```python
from build123d import *

# Parameters (mm, degrees)
SKETCH021_W             = 51.5
SKETCH021_H             = 3
SKETCH021_W_2           = 3
SKETCH021_H_2           = 51.5
PAD014_DEPTH            = 1.6
SKETCH022_R             = 3
PAD015_DEPTH            = 2.6
HOLE_D                  = 3.4
HOLE_DEPTH              = 25
HOLE_CSINK_D            = 6.7
HOLE_CSINK_ANGLE        = 90
BODY005_PLACEMENT_ANGLE = 180


with BuildPart() as part:
    # Sketch021 → Pad014 (new body)
    with BuildSketch(Plane.XY):
        with BuildLine():
            ThreePointArc((-43, 41), (-46.535534, 39.535534), (-48, 36))
            Line((-48, -36), (-48, 36))
            ThreePointArc((-48, -36), (-46.535534, -39.535534), (-43, -41))
            Line((43, -41), (-43, -41))
            ThreePointArc((43, -41), (46.535534, -39.535534), (48, -36))
            Line((48, 36), (48, -36))
            ThreePointArc((48, 36), (46.535534, 39.535534), (43, 41))
            Line((-43, 41), (43, 41))
        make_face()
        with Locations((0, 22)):
            Rectangle(SKETCH021_W, SKETCH021_H, mode=Mode.SUBTRACT)
        with Locations((0, -22)):
            Rectangle(SKETCH021_W, SKETCH021_H, mode=Mode.SUBTRACT)
        with Locations((-36.5, 0)):
            Rectangle(SKETCH021_W_2, SKETCH021_H_2, mode=Mode.SUBTRACT)
        with Locations((36.5, 0)):
            Rectangle(SKETCH021_W_2, SKETCH021_H_2, mode=Mode.SUBTRACT)
    extrude(amount=PAD014_DEPTH)

    # Sketch022 → Pad015 (join)
    with BuildSketch(Plane.XY):
        with Locations((-44, 37)):
            Circle(SKETCH022_R)
        with Locations((12, 37)):
            Circle(SKETCH022_R)
        with Locations((44, 37)):
            Circle(SKETCH022_R)
        with Locations((44, -37)):
            Circle(SKETCH022_R)
        with Locations((12, -37)):
            Circle(SKETCH022_R)
        with Locations((-44, -37)):
            Circle(SKETCH022_R)
    extrude(amount=PAD015_DEPTH)

    # Hole
    with Locations(Plane(origin=(0, 0, 0), x_dir=(1, 0, 0), z_dir=(0, 0, -1))):
        with Locations((-44, -37), (12, -37), (44, -37), (44, 37), (12, 37), (-44, 37)):
            CounterSinkHole(HOLE_D / 2, HOLE_CSINK_D / 2, depth=HOLE_DEPTH, counter_sink_angle=HOLE_CSINK_ANGLE)


with BuildPart() as part_1:
    # Body005 placement: moved
    add(part.part.moved(Location((0, 0, 80.3))).rotate(Axis((0, 0, 80.3), (1, 0, 0)), BODY005_PLACEMENT_ANGLE))


solid = part_1.part
```
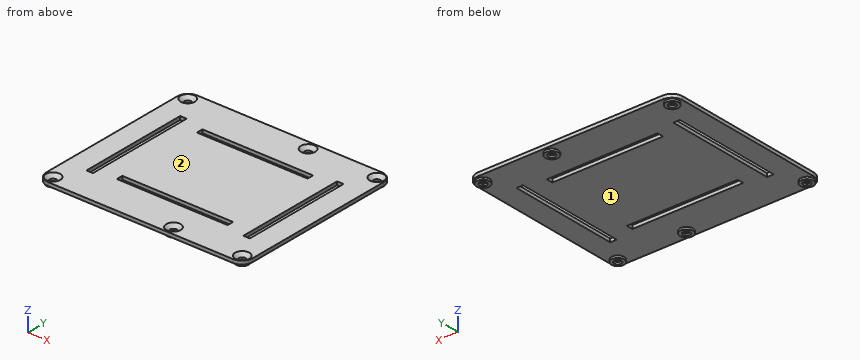
Part model, mm, in its own coordinate system. Face numbers are marked on the shaded views. Round coordinates to 2 decimals unless told otherwise and drop trailing zeros. Loops run counter-clockwise (first coordinate to the right, second up) from the corner with the lowest first, then second, coordinate; pieces in that order, holes last.
Item 1: Cut at A-A, the plane x = -14.5. Give the cut face in (y, z).
Item 2: Cut at B-B, the plane y = -9. Give the cut face in (x, z), then the cut area to 3 significant figures.
Item 3: Drill centre lines: line 1 (X direction, y = -37, z = 78); line 2 (Y direction, x = -2, z = 79.5); line 3 (X direction, y = -11, z = 78.8). Where is each one in solid material? Low to high.
Item 4: Cut at D-D, the plane y = -31. Give the cut face in (x, z).
Item 5: Drop flat-ended pins along their axis: P1, Ø4.5, axis at x = 12, y = 37, coming from the -Z side; P2, Ø3, axis at x = -16, y = 2, coming from the -Z side; P3, Ø4.5, axis at x = -44, y = -37, coming from the +Z side. Give the stop position or say it passes through.
Item 6: Cut at C-C, the plane x = 12. State how many separate pieces and enclosed holes the cut face has, then the cut area to 3 significant figures.
Item 7: Mould opens along X. For the marked faces 1 and 2 say: +X half, -X half, draft (parallel to the pull), parting line (faces both ways), or undercut.
A:
1. outline: (-41, 78.7) - (-23.5, 78.7) - (-23.5, 80.3) - (-41, 80.3) - close; (-20.5, 78.7) - (20.5, 78.7) - (20.5, 80.3) - (-20.5, 80.3) - close; (23.5, 78.7) - (41, 78.7) - (41, 80.3) - (23.5, 80.3) - close
2. outline: (-48, 78.7) - (-38, 78.7) - (-38, 80.3) - (-48, 80.3) - close; (-35, 78.7) - (35, 78.7) - (35, 80.3) - (-35, 80.3) - close; (38, 78.7) - (48, 78.7) - (48, 80.3) - (38, 80.3) - close
2. area: 144 mm2
3. line 1: x = -47 to -45.7, -42.3 to -41, 9 to 10.3, 13.7 to 15, 41 to 42.3, 45.7 to 47
3. line 2: y = -41 to -23.5, -20.5 to 20.5, 23.5 to 41
3. line 3: x = -48 to -38, -35 to 35, 38 to 48
4. outline: (-48, 78.7) - (48, 78.7) - (48, 80.3) - (-48, 80.3) - close
5. P1: stops at z = 77.7
5. P2: stops at z = 78.7
5. P3: stops at z = 79.2
6. separate pieces: 5
6. enclosed holes: 0
6. area: 110 mm2
7. face 1: undercut
7. face 2: draft
